```python
from build123d import *

# Parameters (mm, degrees)
F1_DEPTH = 3.175


with BuildPart() as f1:
    # F0 (on Front) → F1 (new body)
    with BuildSketch(Plane.XZ):
        Polygon((-113.5953023911, 200.9700069427), (-253.2953023911, 200.9700069427), (-253.2953023911, 188.2700069427), (-256.4703023911, 188.2700069427), (-256.4703023911, 175.5700069427), (-253.2953023911, 175.5700069427), (-253.2953023911, 162.8700069427), (-256.4703023911, 162.8700069427), (-256.4703023911, 150.1700069427), (-253.2953023911, 150.1700069427), (-253.2953023911, 137.4700069427), (-234.2453023911, 137.4700069427), (-234.2453023911, 134.2950069427), (-221.5453023911, 134.2950069427), (-221.5453023911, 137.4700069427), (-189.7953023911, 137.4700069427), (-189.7953023911, 134.2950069427), (-177.0953023911, 134.2950069427), (-177.0953023911, 137.4700069427), (-145.3453023911, 137.4700069427), (-145.3453023911, 134.2950069427), (-132.6453023911, 134.2950069427), (-132.6453023911, 137.4700069427), (-113.5953023911, 137.4700069427), (-113.5953023911, 150.1700069427), (-110.4203023911, 150.1700069427), (-110.4203023911, 162.8700069427), (-113.5953023911, 162.8700069427), (-113.5953023911, 175.5700069427), (-110.4203023911, 175.5700069427), (-110.4203023911, 188.2700069427), (-113.5953023911, 188.2700069427), align=None)
        with BuildLine():
            ThreePointArc((-231.0703023911, 146.2012569427), (-229.3865043684, 145.5038049654), (-228.6890523911, 143.8200069427))
            ThreePointArc((-228.6890523911, 143.8200069427), (-232.7541004138, 142.13620892), (-231.0703023911, 146.2012569427))
        make_face(mode=Mode.SUBTRACT)
    extrude(amount=F1_DEPTH)


solid = f1.part
```
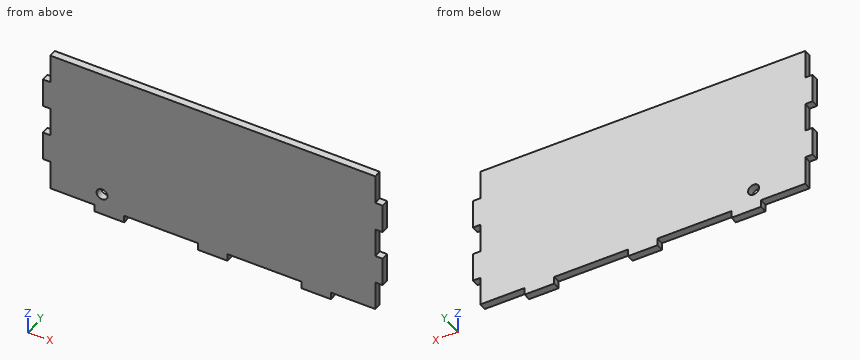
Geometry: final body of the model. Coordinates: model frame, mm. Round coordinates to 2 decimals unless told otherwise and drop trailing zeros. Write each loop counter-clockwise with the first axis right and the second up, starting at its lowest first coordinate (ties: lowest second). Pieces come first, ordered by that corner, then holes. Notation, with made-up numbers: (-12.75, 51) -> (43.25, 51) arc R25 cw to (43.25, 79) -> close; hole circle Ø8 at (-25.5, -29). An arc over 180 degrees is marked (long way). Return JSON: item names as keys, results as strings.
Q1. First-contact query: pin 1 Ø1 at (x, y) = (-255.5, -1) entering from -Z; pin 2 Ø1.6 at (x, y) = (-241, -2) entering from -Z; pin 3 Ø1 at (x, y) = (-112, -2) entering from +Z. Flat tips, straight axial feed; report the tip coordinate or a pass-through.
From the geometry:
{"pin 1": "z = 150.17", "pin 2": "z = 137.47", "pin 3": "z = 188.27"}
Q2. Section B-B on z = 194. Return the cut outline in (x, y) (3 decimals).
From the geometry:
{"outline": "(-253.295, -3.175) -> (-113.595, -3.175) -> (-113.595, 0) -> (-253.295, 0) -> close"}
Q3. Ray query, line 1 (X direction, y = -1.85, z = 163.5); line 2 (Z direction, x = -170.5, y = -1.95); line 3 (Z direction, x = -232.5, y = -2.05) (3 decimals). Return the intervals inside material, ascending.
From the geometry:
{"line 1": "-253.3 to -113.6", "line 2": "137.47 to 200.97", "line 3": "134.295 to 141.916, 145.724 to 200.97"}
Q4. Section C-C on x = -168. Return the cut outline in (y, z) (3 decimals).
From the geometry:
{"outline": "(-3.175, 137.47) -> (0, 137.47) -> (0, 200.97) -> (-3.175, 200.97) -> close"}
